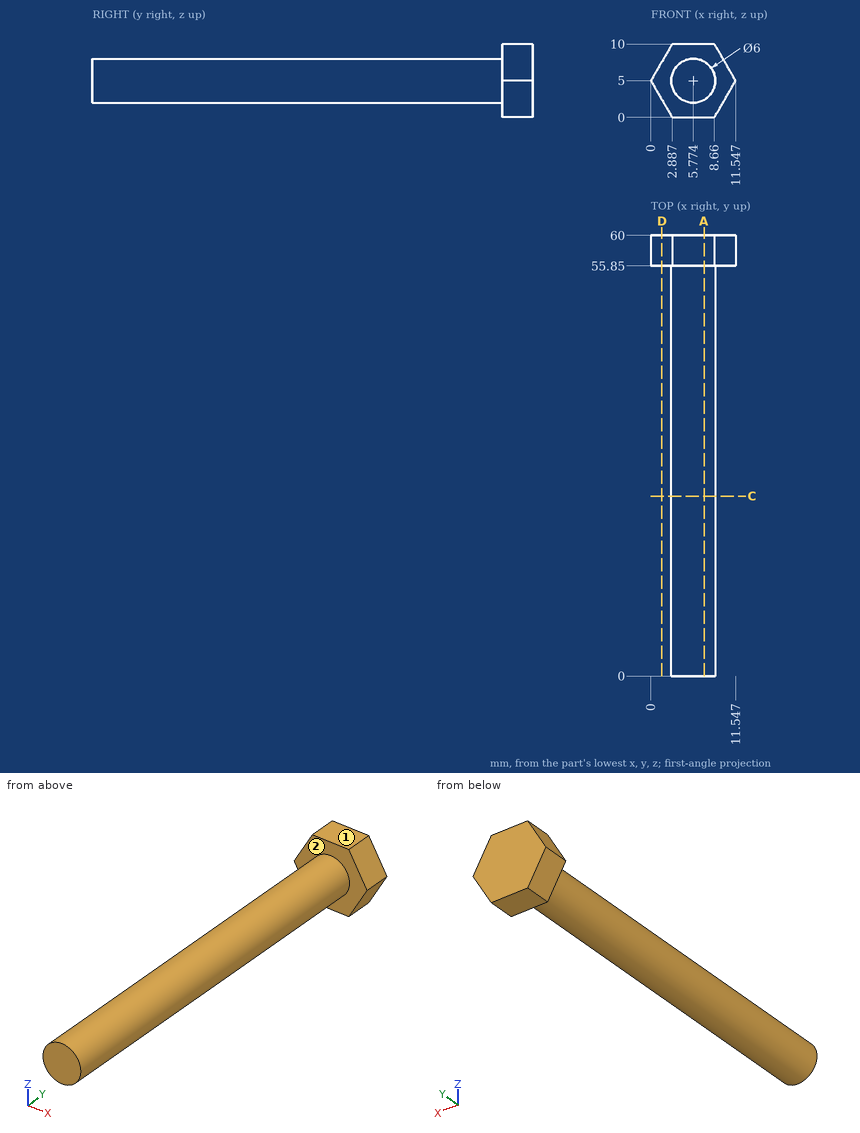
Check sheet for the drawn part. Datum: minimum x, y, z corner. Units: mm. A direction names the side the tool comes from. Coordinates: 2 decimals unless noted, no trailing zeros. Loops run counter-clockwise (first coordinate to the right, second up) from the corner with the lowest first, then second, coordinate; pieces in that order, holes last. Notation, with made-up numbers: (32, -32.5) -> (42, -32.5) arc R13 cw to (42, -7.5) -> close; hole circle Ø4 at (39, -21). An arc over 180 degrees is marked (long way). Answer as CSV lines item,"result".
1) Cross-section at D-D, the plane x = 1.5. Record the cut outline in (y, z).
Found:
outline,"(55.85, 2.4) -> (60, 2.4) -> (60, 7.6) -> (55.85, 7.6) -> close"
2) Cross-section at C-C, the plane y = 24.5. Record the cut outline in (x, z).
Found:
outline,"circle Ø6 at (5.77, 5)"
3) Tool access check on the marked faces 1 and 2. Record the directions out of +Z, -Z, +X, -X, +Y, -Y that give a thin tool (end or side, any length) a straight path to the whole face; none if there is none.
Found:
face 1,"+Z, +X, -X, +Y, -Y"
face 2,"-Y"
4) Depth check by flat-ended pin: pin 1 (5 mm diameter, centred on y = 9, z = 3.5, fed in from -X); pin 2 (2 mm diameter, centred on x = 5, y = 23, fed in from +Z). Enter the tip coordinate at first touch or a pass-through.
Found:
pin 1,"stops at x = 2.77"
pin 2,"stops at z = 8"
5) Thickness scan on L1, parallel to Y at x = 2.5, z = 6.5; L2, parallel to X at y = 3, z = 7.75 (1 decimal); L3, parallel to X at y = 45, z = 6.25 (1 decimal). Record the ranges inside material, lowest first. Write a range as from..to.
Found:
L1,"y = 55.85..60"
L2,"x = 4.6..7"
L3,"x = 3..8.5"
6) Cross-section at A-A, the plane x = 7.25. Record the cut outline in (y, z), then the cut area to 3 significant figures.
Found:
outline,"(0, 2.39) -> (55.85, 2.39) -> (55.85, 0) -> (60, 0) -> (60, 10) -> (55.85, 10) -> (55.85, 7.61) -> (0, 7.61) -> close"
area,"333 mm2"
